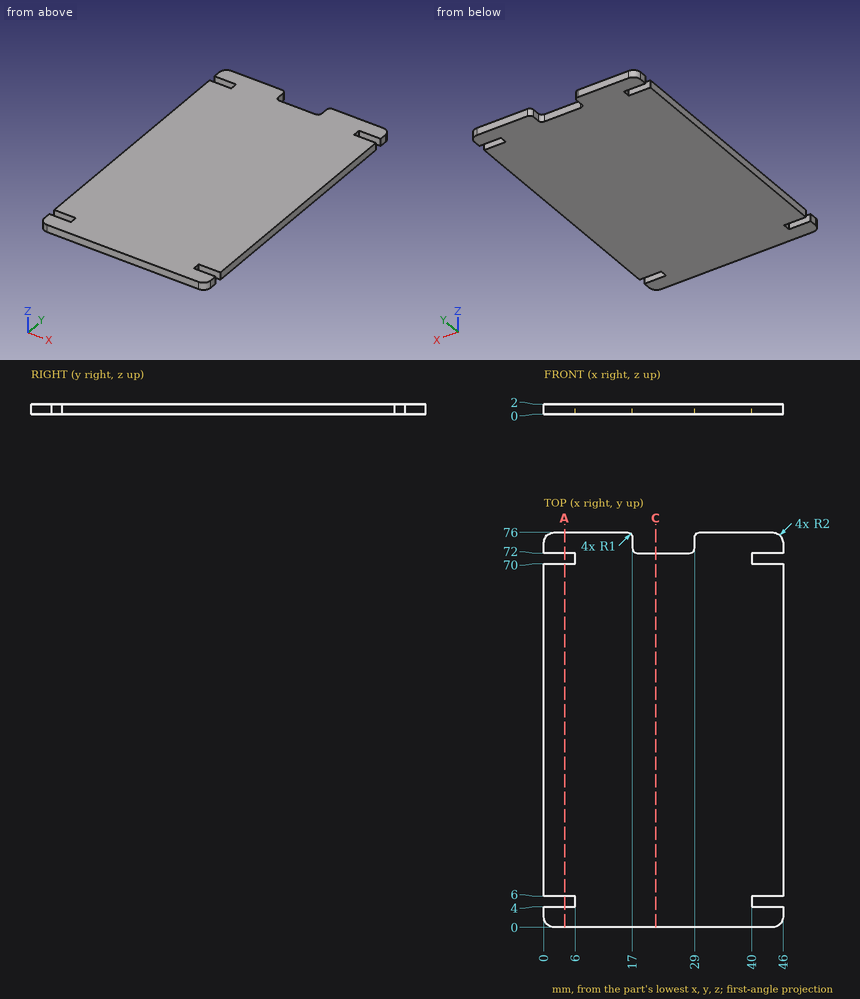
Print and shaded views of the part. All mm, measured from the part's lowest x, y and z. Coordinates: 2 decimals unless noted, no trailing zeros. Order: outer loops, then holes, each group sorted by start corner. A loop starts at its lowest first (then second) coordinate and runs counter-clockwise, first axis right, second up. Notation, with made-up numbers: (9.25, 54) -> (25.25, 54) arc R30 cw to (25.25, 90) -> close; hole circle Ø6 at (53, 75). An arc over 180 degrees is marked (long way). Use one line per item in the form item = value. Start each with the question number.
1) Drill centre lines: L1, parallel to Y at x = 2, z = 1.3; L2, parallel to Y at x = 19.5, z = 0.6. Where is each one in solid material? Low to high. Write a range as [from, to].
2) Band-saw the part on A-A on x = 4. Give the cut face in (y, z).
3) Band-saw the part on C-C on x = 21.5. Give the cut face in (y, z), then the cut area to 3 significant figures.
4) Drop flat-ended pins along their axis: pin 1 (0.6 mm diameter, centred on y = 5, z = 1, fed in from -X); pin 2 (4 mm diameter, centred on x = 7, y = 8, fed in from -Z); pin 3 (1 mm diameter, centred on y = 71, z = 1.5, fed in from +X). Give the stop position or say it passes through.
Entries:
q1.L1 = [0, 4], [6, 70], [72, 76]
q1.L2 = [0, 72]
q2.outline = (0, 0) -> (4, 0) -> (4, 2) -> (0, 2) -> close; (6, 0) -> (70, 0) -> (70, 2) -> (6, 2) -> close; (72, 0) -> (76, 0) -> (76, 2) -> (72, 2) -> close
q3.outline = (0, 0) -> (72, 0) -> (72, 2) -> (0, 2) -> close
q3.area = 144 mm2
q4.pin_1 = 6
q4.pin_2 = 0
q4.pin_3 = 40
